Geometry check sheet. Reference: the model listing, model coordinates, mm. A direction names the side the tool comes from. Coordinates: 2 decimals unless noted, no trailing zeros. Loops run counter-clockwise (first coordinate to the right, second up) from the corner with the lowest first, then second, coordinate; pieces in that order, holes last. Notation, with made-up numbers: (60, -6) - (113, -6) arc R9 cw to (113, 9) - close; hole circle Ø8 at (-31.5, 17). An arc over 180 degrees is marked (long way). Write each question's results on one line, items separated by ' | '. Start each with the question number.
(1) Go/stop test with a flat-tipped pin: pin 1 Ø3 at (x, z) = (-14.5, -44) entering from +Y. Record where the tip stops, or that it passes through.
(2) Sectioned sample at A-A (y = 13.25). Enter the section's corners in (x, z), plus the area to 3 significant figures.
(3) Sectioned sample at B-B (x = -5.75). Enter the section's corners in (y, z), plus the area to 3 significant figures.
(4) Material ranges on probe 1 along Y at (x, z) = (-17.5, -42); probe 2 along Z at (x, y) = (-17, 15); probe 3 along X at (y, z) = (16.5, -59.5), recorded low to high.
(5) Mould release check, pull along Z, two halves, no side actions. Record for faces 1 (the face through (-31.27, 5, -57)), 2 (the face through (-16, 5, -81.759)), 3 (the face through (-13.961, 12.712, -61.717)): pulls with the +Z half, pulls with the -Z half, needs draft (parallel to the pull), parting line crosses it, or undercut.
(6) Access from +Z, -Z, +X, -X, +Y, -Y to the whole of each face (thin tool, end or side, straight path). Record for faces 4 (the face through (-15.12, 12.71, -78.48)), 5 (the face through (-16.3, 17.5, -45.3)).
Autodesk Inventor part; units mm, degrees
ref_plane "YZ Plane" through (0, 0, 0) normal (1, 0, 0) x (0, 1, 0)
ref_plane "XZ Plane" through (0, 0, 0) normal (0, 1, 0) x (-1, 0, 0)
ref_plane "XY Plane" through (0, 0, 0) normal (0, 0, 1) x (1, 0, 0)
sketch "Skizze1" plane through (0, 0, 0) normal (0, 1, 0) x (-1, 0, 0)
  line L0 (31.2704, -31.759) -> (1.2704, -31.759)
  line L1 (1.2704, -31.759) -> (1.2704, -81.759)
  line L2 (1.2704, -81.759) -> (31.2704, -81.759)
  line L3 (31.2704, -81.759) -> (31.2704, -31.759)
  point P0 (0, 0)
  dimension "d0" = 50
  dimension "d1" = 30
extrude "Extrusion1" add sketch "Skizze1" along normal blind 10
sketch "Skizze2" plane through (0, 10, 0) normal (0, 1, 0) x (1, 0, 0)
  circle A0 centre (-16.2704, 37.259) radius 2.5
  circle A1 centre (-16.2704, 60.759) radius 2.5
  circle A2 centre (-16.2704, 76.259) radius 2.5
  circle A3 centre (-16.2704, 45.259) radius 2.5
  circle A4 centre (-16.2704, 52.759) radius 2.5
  circle A5 centre (-16.2704, 68.259) radius 2.5
  line L0 (-31.2704, 81.759) -> (-31.2704, 31.759)
  line L1 (-31.2704, 31.759) -> (-1.2704, 31.759)
  line L2 (-1.2704, 81.759) -> (-31.2704, 81.759)
  point P0 (0, 0)
  dimension "d4" = 5
  dimension "d5" = 5
  dimension "d6" = 5
  dimension "d7" = 5
  dimension "d10" = 5
  dimension "d11" = 5
  dimension "d12" = 15
  dimension "d13" = 15
  dimension "d14" = 15
  dimension "d15" = 15
  dimension "d16" = 15
  dimension "d17" = 15
  dimension "d18" = 8
  dimension "d19" = 8
  dimension "d20" = 8
  dimension "d22" = 5.5
  dimension "d23" = 5.5
  dimension "d24" = 21
extrude "Extrusion2" add sketch "Skizze2" along normal blind 7.5
fillet "Rundung1" radius 2 6 edges at (-18.7704, 17.5, -37.259) (-18.7704, 17.5, -45.259) (-18.7704, 17.5, -52.759) (-18.7704, 17.5, -60.759) (-18.7704, 17.5, -68.259) (-18.7704, 17.5, -76.259)
properties part number "Linien-Sensor" material "Nylon 6/6"
Outcome:
1) pin 1: stops at y = 17.49
2) outline: circle Ø5 at (-16.27, -76.26); circle Ø5 at (-16.27, -68.26); circle Ø5 at (-16.27, -60.76); circle Ø5 at (-16.27, -52.76); circle Ø5 at (-16.27, -45.26); circle Ø5 at (-16.27, -37.26) | area: 118 mm2
3) outline: (0, -81.76) - (10, -81.76) - (10, -31.76) - (0, -31.76) - close | area: 500 mm2
4) probe 1: y = 0 to 10 | probe 2: z = -78.65 to -73.87, -70.65 to -65.87, -63.15 to -58.37, -55.15 to -50.37, -47.65 to -42.87, -39.65 to -34.87 | probe 3: x = -18.11 to -14.43
5) face 1: needs draft | face 2: pulls with the -Z half | face 3: undercut
6) face 4: +Y | face 5: +Z, -Z, +X, -X, +Y
